Geometry: see drawing. Coordinates: mm, zero at the bounding-box minimum. Give positions to 0.01 mm unless a question says otherwise; leave off trailing zeros. Loops run counter-clockwise (first coordinate to the right, second up) from the corner with the lowest first, then second, coordinate; pieces in that order, holes last. Notation, with made-up numbers: (15, 6) -> (40, 6) arc R26 ccw to (40, 24) -> close; hole circle Ø1 at (-21, -31.75). An arc over 180 degrees is marked (long way). Return JSON: item names as keys, results as strings. Group by question number.
(1) Cut plane C-C on z = 614. Return loops of the section in (x, y), then the cut area to 3 significant figures.
(2) Cut plane A-A on y = 63.5. Return loops of the section in (x, z).
(3) Cut plane B-B on x = 24. Return loops of the section in (y, z), then the cut area to 3 significant figures.
(4) Ray query, line 1 (Z direction, x = 19, y = 34); line 2 (Y direction, x = 21.5, z = 330.5). Return the intervals inside material, ascending. Write a range as from..to.
(5) Pin query (flat end, axial travel): pin 1 (10 mm diameter, centred on x = 25, z = 88, fed in from -Y); pin 2 (1.5 mm diameter, centred on x = 26, y = 45, fed in from +Z); pin 3 (14.5 mm diameter, centred on x = 13, z = 641, fed in from +Y); pin 4 (1.5 mm diameter, centred on x = 9.5, y = 40, fed in from -Z). Return the tip coordinate at first contact, or that it passes through.
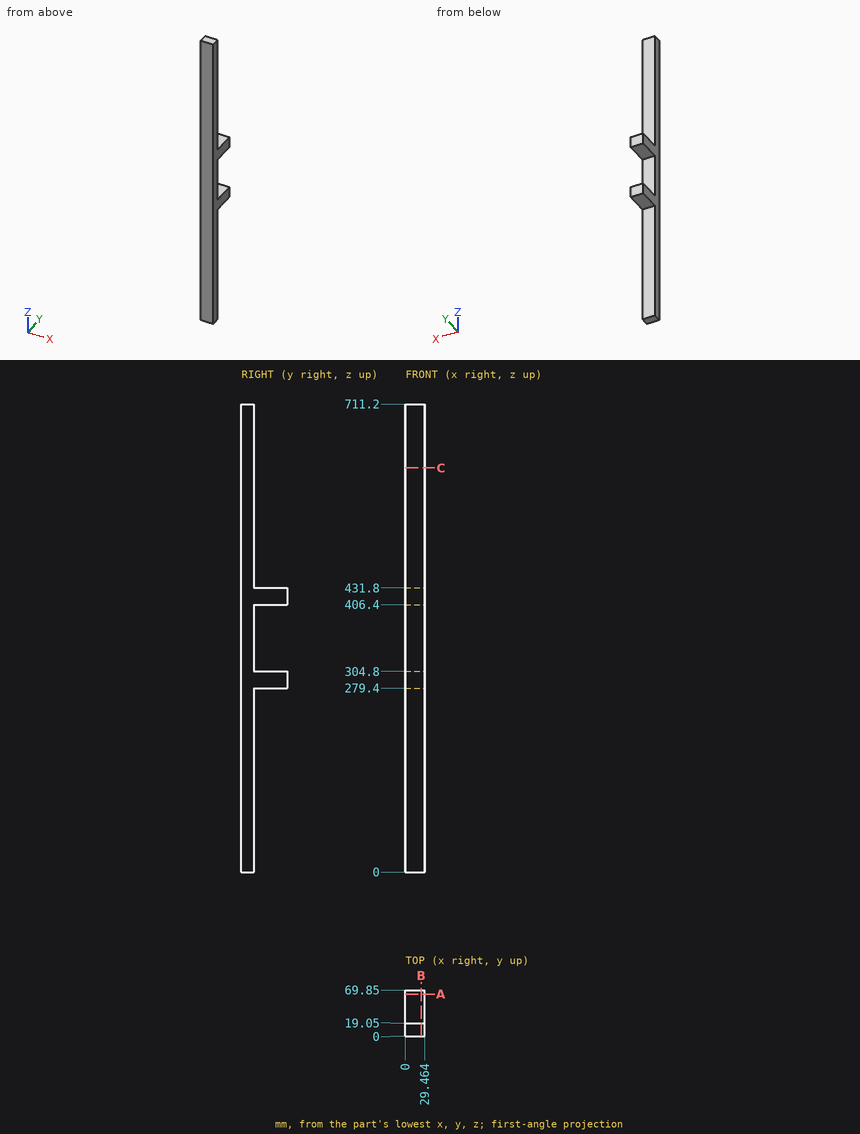
Answers:
{
 "1": {"outline": "(0, 0) -> (29.46, 0) -> (29.46, 19.05) -> (0, 19.05) -> close", "area": "561 mm²"},
 "2": {"outline": "(0, 279.4) -> (29.46, 279.4) -> (29.46, 304.8) -> (0, 304.8) -> close; (0, 406.4) -> (29.46, 406.4) -> (29.46, 431.8) -> (0, 431.8) -> close"},
 "3": {"outline": "(0, 0) -> (19.05, 0) -> (19.05, 279.4) -> (69.85, 279.4) -> (69.85, 304.8) -> (19.05, 304.8) -> (19.05, 406.4) -> (69.85, 406.4) -> (69.85, 431.8) -> (19.05, 431.8) -> (19.05, 711.2) -> (0, 711.2) -> close", "area": "16,100 mm²"},
 "4": {"line 1": "279.4..304.8, 406.4..431.8", "line 2": "0..19.05"},
 "5": {"pin 1": "y = 0", "pin 2": "z = 431.8", "pin 3": "y = 19.05", "pin 4": "z = 279.4"}
}
